Model file for the job. Use its own axes, mm. Round coordinates to 2 decimals unless told otherwise and drop trailing zeros. Loops run counter-clockwise (first coordinate to the right, second up) from the corner with the lowest first, then second, coordinate; pieces in that order, holes last. Notation, with made-up numbers: (21, 70) - (63, 70) arc R25 cw to (63, 94) - close; hole circle Ø6 at (-27, 16). An arc over 180 degrees is marked (long way). Use one line per item in the form item = value.
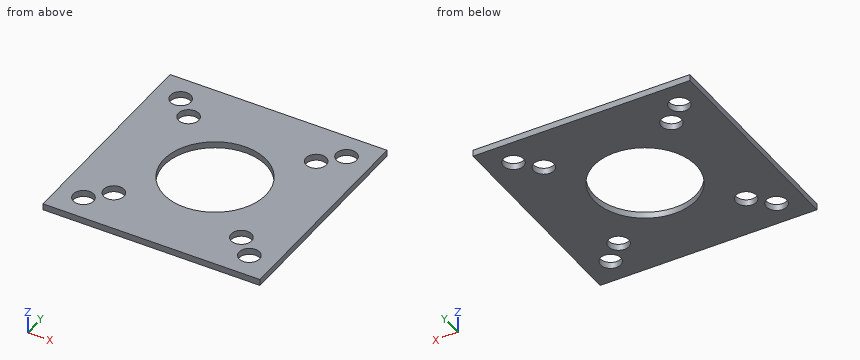
from build123d import *

# Parameters (mm, degrees)
SKETCH_W        = 34
SKETCH_H        = 34
SKETCH_R        = 8
PAD_DEPTH       = 1
SKETCH001_R     = 1.6
POCKET_DEPTH    = 5
SKETCH002_R     = 1.6
POCKET001_DEPTH = 5


with BuildPart() as part:
    # Sketch → Pad (new body)
    with BuildSketch(Plane.XY):
        Rectangle(SKETCH_W, SKETCH_H)
        Circle(SKETCH_R, mode=Mode.SUBTRACT)
    extrude(amount=PAD_DEPTH)

    # Sketch001 (on Face7 of Pad) → Pocket (cut)
    with BuildSketch(Plane.XY.offset(1)):
        with Locations((10, 10)):
            Circle(SKETCH001_R)
        with Locations((10, -10)):
            Circle(SKETCH001_R)
        with Locations((-10, 10)):
            Circle(SKETCH001_R)
        with Locations((-10, -10)):
            Circle(SKETCH001_R)
    extrude(amount=-POCKET_DEPTH, mode=Mode.SUBTRACT)

    # Sketch002 (on Face5 of Pocket) → Pocket001 (cut)
    with BuildSketch(Plane.XY.offset(1)):
        with Locations((-13, 13)):
            Circle(SKETCH002_R)
        with Locations((13, 13)):
            Circle(SKETCH002_R)
        with Locations((-13, -13)):
            Circle(SKETCH002_R)
        with Locations((13, -13)):
            Circle(SKETCH002_R)
    extrude(amount=-POCKET001_DEPTH, mode=Mode.SUBTRACT)


solid = part.part
1. Cut at D-D, the plane z = 0.75. Give the number of separate pieces and of enclosed holes in the cut face, plus the area to 3 significant figures.
Geometry check:
separate_pieces = 1
enclosed_holes = 9
area = 891 mm^2
2. Cut at C-C, the plane y = -6.5. Give the cut face in (x, z).
Geometry check:
outline = (-17, 0) - (-4.66, 0) - (-4.66, 1) - (-17, 1) - close; (4.66, 0) - (17, 0) - (17, 1) - (4.66, 1) - close
3. Cut at A-A, the plane y = -10. Give the cut face in (x, z), plus the area to 3 significant figures.
Geometry check:
outline = (-17, 0) - (-11.6, 0) - (-11.6, 1) - (-17, 1) - close; (-8.4, 0) - (8.4, 0) - (8.4, 1) - (-8.4, 1) - close; (11.6, 0) - (17, 0) - (17, 1) - (11.6, 1) - close
area = 27.6 mm^2
4. Cut at B-B, the plane x = -6. Give the cut face in (y, z).
Geometry check:
outline = (-17, 0) - (-5.29, 0) - (-5.29, 1) - (-17, 1) - close; (5.29, 0) - (17, 0) - (17, 1) - (5.29, 1) - close
5. Wall check: probe 1 along Y at (x, z) = (-10, 0.8); probe 2 along Y at (x, z) = (-13, 0.85); probe 3 along X at (y, z) = (-12, 0.3). Give the ranges that are in metal, low to high.
Geometry check:
probe_1 = -17 to -11.6, -8.4 to 8.4, 11.6 to 17
probe_2 = -17 to -14.6, -11.4 to 11.4, 14.6 to 17
probe_3 = -17 to -14.25, -11.75 to 11.75, 14.25 to 17
